Check sheet for the modelled part. Datum: model origin and axes. Units: mm. Face numbers are marked on the shaded views. A direction names the side the tool comes from. Coordinates: 2 decimals unless noted, no trailing zeros. Loops run counter-clockwise (first coordinate to the right, second up) from the corner with the lowest first, then second, coordinate; pieces in that order, holes last. Notation, with made-up numbers: (84.25, 56) - (130.25, 56) arc R16 ccw to (130.25, 61) - close; hole circle Ø6 at (-13, 25.5). An arc over 180 degrees is marked (long way). Use a Markdown table: item, result. Add a question column.
1) Tool access check on the marked faces 1, 2, 3, 4 and 5. Record the directions out of +Z, -Z, +X, -X, +Y, -Y that give a thin tool (end or side, any length) a straight path to the whole face; none if there is none.
2) Draft check along X on the marked faces 6, 7 and 8. Enter one of: pulls with the +X half, pulls with the -X half, needs draft (parallel to the pull), parting line crosses it, or undercut.
3) Thickness scan on line 1 (X direction, y = 28, z = 9); line 2 (X direction, y = 3.9, z = 9); line 3 (X direction, y = 19, z = 0) (3 decimals). Record the ranges inside material, lowest first.
4) Sectioned sample at A-A, the plane x = 0. Enter the section's corners in (y, z) (3 decimals), then the cut area to 3 significant figures.
5) Sectioned sample at B-B, the plane z = -18. Enter the section's corners in (x, y) (3 decimals).
6) Sectioned sample at C-C, the plane y = 29.5. Enter the section's corners in (x, z) (3 decimals).
7) Go/stop test with flat-tipped pins: P1, Ø10, axis at y = 32.5, z = 2, coming from the +X side; P2, Ø7, axis at x = 0, z = -18, coming from the +Y side; P3, Ø2, axis at x = 9.5, y = 5.5, coming from the -Z side. Record where each tip stops, or that it passes through.
8) Sectioned sample at D-D, the plane y = 4. Enter the section's corners in (x, z) (3 decimals).
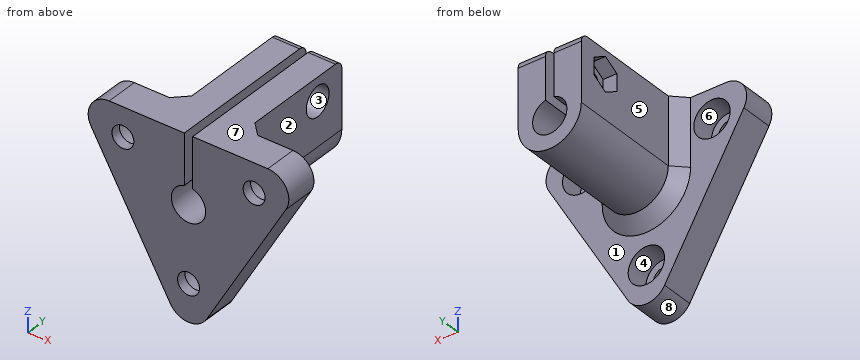
from build123d import *

# Parameters (mm, degrees)
ESQUISSE5_R              = 2.6
BOSS_EXTRU_2_DEPTH       = 7.8
ESQUISSE6_R              = 7.5
BOSS_EXTRU_3_DEPTH       = 30
BOSS_EXTRU_6_START       = -30
BOSS_EXTRU_6_DEPTH       = 30
ESQUISSE14_R             = 4.075
ENL_V_MAT_EXTRU_4_DEPTH  = 57.510382527
ENL_V_MAT_EXTRU_5_DEPTH  = 57.510382527
CONG_2_R                 = 5
ESQUISSE17_R             = 2.075
ENL_V_MAT_EXTRU_6_DEPTH  = 56.917889465
ENL_V_MAT_EXTRU_7_DEPTH  = 3.25
CHANFREIN1_SIZE          = 3
ESQUISSE20_R             = 3.525
ENL_V_MAT_EXTRU_9_DEPTH  = 4.97
CONG_3_R                 = 2
ESQUISSE19_R             = 4.325
ENL_V_MAT_EXTRU_8_DEPTH  = 5.5
ENL_V_MAT_EXTRU_10_DEPTH = 54.291595842


with BuildPart() as part:
    # Esquisse5 → Boss.-Extru.2 (new body)
    with BuildSketch(Plane(origin=(0, 0, 0), x_dir=(1, 0, 0), z_dir=(0, 1, 0))):
        Polygon((-27.5, -15.877132403), (27.5, -15.877132403), (0, 31.754264805), align=None)
        with Locations(Location((0, 18, 0), (0, 0, 270))):
            Circle(ESQUISSE5_R, mode=Mode.SUBTRACT)
        with Locations(Location((-15.588457268, -9, 0), (0, 0, 270))):
            Circle(ESQUISSE5_R, mode=Mode.SUBTRACT)
        with Locations(Location((15.588457268, -9, 0), (0, 0, 270))):
            Circle(ESQUISSE5_R, mode=Mode.SUBTRACT)
    extrude(amount=BOSS_EXTRU_2_DEPTH)

    # Esquisse6 → Boss.-Extru.3 (add)
    with BuildSketch(Plane(origin=(0, 7.8, 0), x_dir=(1, 0, 0), z_dir=(0, 1, 0))):
        with Locations(Location((0, 0, 0), (0, 0, 270))):
            Circle(ESQUISSE6_R)
    extrude(amount=BOSS_EXTRU_3_DEPTH)

    # Esquisse13 → Boss.-Extru.6 (add)
    with BuildSketch(Plane(origin=(0, 37.8, 0), x_dir=(1, 0, 0), z_dir=(0, 1, 0)).offset(BOSS_EXTRU_6_START)):
        with BuildLine():
            Line((-7.5, 0), (-7.5, -15.877132403))
            Line((-7.5, -15.877132403), (7.5, -15.877132403))
            Line((7.5, -15.877132403), (7.5, 0))
            ThreePointArc((7.5, 0), (0, -7.5), (-7.5, 0))
        make_face()
    extrude(amount=BOSS_EXTRU_6_DEPTH)

    # Esquisse14 → Enlèv. mat.-Extru.4 (cut, through all)
    with BuildSketch(Plane(origin=(0, 37.8, 0), x_dir=(1, 0, 0), z_dir=(0, 1, 0))):
        with Locations(Location((0, 0, 0), (0, 0, 270))):
            Circle(ESQUISSE14_R)
    extrude(amount=-ENL_V_MAT_EXTRU_4_DEPTH, mode=Mode.SUBTRACT)

    # Esquisse15 → Enlèv. mat.-Extru.5 (cut, through all)
    with BuildSketch(Plane(origin=(0, 37.8, 0), x_dir=(1, 0, 0), z_dir=(0, 1, 0))):
        with BuildLine():
            Line((-1, -3.95039555), (-1, -15.877132403))
            Line((-1, -15.877132403), (1, -15.877132403))
            Line((1, -15.877132403), (1, -3.95039555))
            ThreePointArc((1, -3.95039555), (0, -4.075), (-1, -3.95039555))
        make_face()
    extrude(amount=-ENL_V_MAT_EXTRU_5_DEPTH, mode=Mode.SUBTRACT)

    # Congé2
    cong_2_edges = [part.edges().sort_by_distance(p)[0] for p in [
        (0, 3.9, -31.754264805),
        (27.5, 3.9, 15.877132403),
        (-27.5, 3.9, 15.877132403),
    ]]
    fillet(cong_2_edges, radius=CONG_2_R)

    # Esquisse17 → Enlèv. mat.-Extru.6 (cut, through all)
    with BuildSketch(Plane(origin=(7.5, 0, 0), x_dir=(0, 0, -1), z_dir=(1, 0, 0))):
        with Locations((-10.377132403, 30.3)):
            Circle(ESQUISSE17_R)
    extrude(amount=-ENL_V_MAT_EXTRU_6_DEPTH, mode=Mode.SUBTRACT)

    # Esquisse18 → Enlèv. mat.-Extru.7 (cut)
    with BuildSketch(Plane.ZY.offset(7.5)):
        Polygon((12.412292102, 33.825), (8.341972704, 33.825), (6.306813005, 30.3), (8.341972704, 26.775), (12.412292102, 26.775), (14.447451801, 30.3), align=None)
    extrude(amount=-ENL_V_MAT_EXTRU_7_DEPTH, mode=Mode.SUBTRACT)

    # Chanfrein1
    chanfrein1_edges = [part.edges().sort_by_distance(p)[0] for p in [
        (0, 7.8, -7.5),
        (7.5, 7.8, 7.938566201),
        (-7.5, 7.8, 7.938566201),
    ]]
    chamfer(chanfrein1_edges, length=CHANFREIN1_SIZE)

    # Esquisse20 → Enlèv. mat.-Extru.9 (cut)
    with BuildSketch(Plane(origin=(7.5, 0, 0), x_dir=(0, 0, -1), z_dir=(1, 0, 0))):
        with Locations((-10.377132403, 30.3)):
            Circle(ESQUISSE20_R)
    extrude(amount=-ENL_V_MAT_EXTRU_9_DEPTH, mode=Mode.SUBTRACT)

    # Congé3
    cong_3_edges = [part.edges().sort_by_distance(p)[0] for p in [
        (-4.25, 37.8, 15.877132403),
        (4.25, 37.8, 15.877132403),
    ]]
    fillet(cong_3_edges, radius=CONG_3_R)

    # Esquisse19 → Enlèv. mat.-Extru.8 (cut)
    with BuildSketch(Plane(origin=(0, 7.8, 0), x_dir=(1, 0, 0), z_dir=(0, 1, 0))):
        with Locations(Location((0, 18, 0), (0, 0, 270))):
            Circle(ESQUISSE19_R)
        with Locations(Location((-15.588457268, -9, 0), (0, 0, 270))):
            Circle(ESQUISSE19_R)
        with Locations(Location((15.588457268, -9, 0), (0, 0, 270))):
            Circle(ESQUISSE19_R)
    extrude(amount=-ENL_V_MAT_EXTRU_8_DEPTH, mode=Mode.SUBTRACT)

    # Esquisse21 → Enlèv. mat.-Extru.10 (cut, through all)
    with BuildSketch(Plane(origin=(2.53, 0, 0), x_dir=(0, 0, -1), z_dir=(1, 0, 0))):
        Polygon((-11.336300266, 32.140005981), (-10.377132403, 32.640005981), (-9.417964539, 32.140005981), align=None)
    extrude(amount=-ENL_V_MAT_EXTRU_10_DEPTH, mode=Mode.SUBTRACT)


solid = part.part
Solved:
| question | item | result |
|---|---|---|
| 1 | face 1 | -Z, +Y |
| 1 | face 2 | +Z, -Z, +X, +Y |
| 1 | face 3 | +X |
| 1 | face 4 | +Y |
| 1 | face 5 | +Z, -Z, -X, +Y |
| 2 | face 6 | undercut |
| 2 | face 7 | needs draft |
| 2 | face 8 | parting line crosses it |
| 3 | line 1 | x = -4.25 to -1, 1 to 2.53 |
| 3 | line 2 | x = -23.47 to -19.91, -11.26 to -1, 1 to 11.26, 19.91 to 23.47 |
| 3 | line 3 | x = -7.5 to -4.075, 4.075 to 7.5 |
| 4 | outline | (0, -26.754) - (7.8, -26.754) - (7.8, -22.325) - (2.3, -22.325) - (2.3, -20.6) - (0, -20.6) - close; (0, -15.4) - (2.3, -15.4) - (2.3, -13.675) - (7.8, -13.675) - (7.8, -10.5) - (10.8, -7.5) - (37.8, -7.5) - (37.8, -4.075) - (0, -4.075) - close |
| 4 | area | 225 mm2 |
| 5 | outline | (-7.941, 0) - (-2.6, 0) - (-2.6, 2.3) - (-4.325, 2.3) - (-4.325, 7.8) - (-7.941, 7.8) - close; (2.6, 0) - (7.941, 0) - (7.941, 7.8) - (4.325, 7.8) - (4.325, 2.3) - (2.6, 2.3) - close |
| 6 | outline | (-7.5, 0) arc R7.5 ccw to (7.5, 0) - (7.5, 6.944) - (2.53, 6.944) - (2.53, 8.463) - (1, 8.463) - (1, 3.95) arc R4.075 cw (long way) to (-1, 3.95) - (-1, 8.463) - (-4.25, 8.463) - (-4.25, 6.769) - (-7.5, 6.769) - close; (-7.5, 13.986) - (-4.25, 13.986) - (-4.25, 12.292) - (-1, 12.292) - (-1, 15.877) - (-7.5, 15.877) - close; (1, 12.292) - (2.53, 12.292) - (2.53, 13.81) - (7.5, 13.81) - (7.5, 15.877) - (1, 15.877) - close |
| 7 | P1 | stops at x = 7.5 |
| 7 | P2 | stops at y = 2.3 |
| 7 | P3 | stops at z = -17.03 |
| 8 | outline | (-23.17, 8.377) - (-4.33, -24.254) arc R5 ccw to (4.33, -24.254) - (23.17, 8.377) arc R5 ccw to (18.84, 15.877) - (1, 15.877) - (1, 3.95) arc R4.075 cw (long way) to (-1, 3.95) - (-1, 15.877) - (-18.84, 15.877) arc R5 ccw to start; hole circle Ø8.65 at (-15.588, 9); hole circle Ø8.65 at (0, -18); hole circle Ø8.65 at (15.588, 9) |
